Autodesk Inventor part; units mm, degrees
ref_plane "YZ Plane" through (0, 0, 0) normal (1, 0, 0) x (0, 1, 0)
ref_plane "XZ Plane" through (0, 0, 0) normal (0, 1, 0) x (-1, 0, 0)
ref_plane "XY Plane" through (0, 0, 0) normal (0, 0, 1) x (1, 0, 0)
sketch "Boceto1" plane through (0, 0, 0) normal (0, 0, 1) x (1, 0, 0)
  line L0 (0, 0) -> (52, 0)
  line L1 (52, 0) -> (52, 60)
  line L2 (0, 60) -> (0, 0)
  line L3 (26, 63) -> (21, 63)
  line L4 (21, 63) -> (21, 60)
  line L5 (26, 63) -> (31, 63)
  line L6 (31, 63) -> (31, 60)
  line L7 (52, 60) -> (31, 60)
  line L8 (21, 60) -> (0, 60)
  dimension "d0" = 52
  dimension "d1" = 60
extrude "Extrusión1" add sketch "Boceto1" along normal blind 5
properties part number "bateria" material "Aluminum 6061"
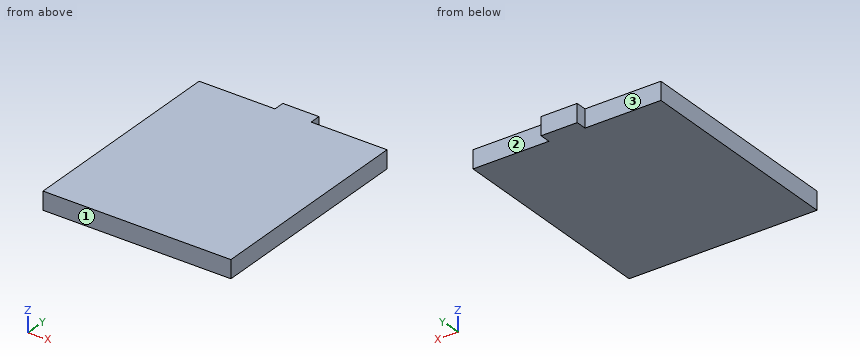
Could you check a few things on this model? Use its own coordinates, in mm. Face numbers are marked on the shaded views. A direction names the side the tool comes from. Coordinates: 2 decimals unless noted, no trailing zeros. Write each loop counter-clockwise with the first axis right and the second up, starting at its lowest first coordinate (ties: lowest second). Pieces come first, ordered by that corner, then holes. Notation, with made-up numbers: (31, 38) -> (35, 38) arc R14 ccw to (35, 57) -> close; hole circle Ø7 at (17.5, 61.25). An arc over 180 degrees is marked (long way). Return JSON: item names as keys, results as strings.
(1) Which directions (+Z, -Z, +X, -X, +Y, -Y) give clear straight access to the entire face, cutting with the end or side of a thin tool? Please do the marked faces 1, 2 and 3.
Numbers:
{"face 1": "+Z, -Z, +X, -X, -Y", "face 2": "+Z, -Z, +X, +Y", "face 3": "+Z, -Z, -X, +Y"}
(2) I'm going to push flat-ended pins straight in: pin 1 (2 mm diameter, centred on x = 39, y = 52, fed in from -Z); pin 2 (1.5 mm diameter, centred on x = 5.5, z = 2, fed in from +Y); pin 3 (2.5 mm diameter, centred on y = 62, z = 3.5, fed in from +X). Where does each tip first touch, or does it pass through?
Numbers:
{"pin 1": "stops at z = 0", "pin 2": "stops at y = 60", "pin 3": "stops at x = 31"}
(3) Imagine slicing it at A-A, the plane z = 1.85. Please give me the cut outline in (x, y).
Numbers:
{"outline": "(0, 0) -> (52, 0) -> (52, 60) -> (31, 60) -> (31, 63) -> (21, 63) -> (21, 60) -> (0, 60) -> close"}
(4) I need wall thicknesses on L1, parallel to Y at x = 47, z = 2.75. Which ranges of the line are inside material? Lowest first, please.
Numbers:
{"L1": "y = 0 to 60"}
(5) Imagine slicing it at B-B, the plane x = 7. Please give me the cut outline in (y, z), then the cut area to 3 significant figures.
Numbers:
{"outline": "(0, 0) -> (60, 0) -> (60, 5) -> (0, 5) -> close", "area": "300 mm2"}
